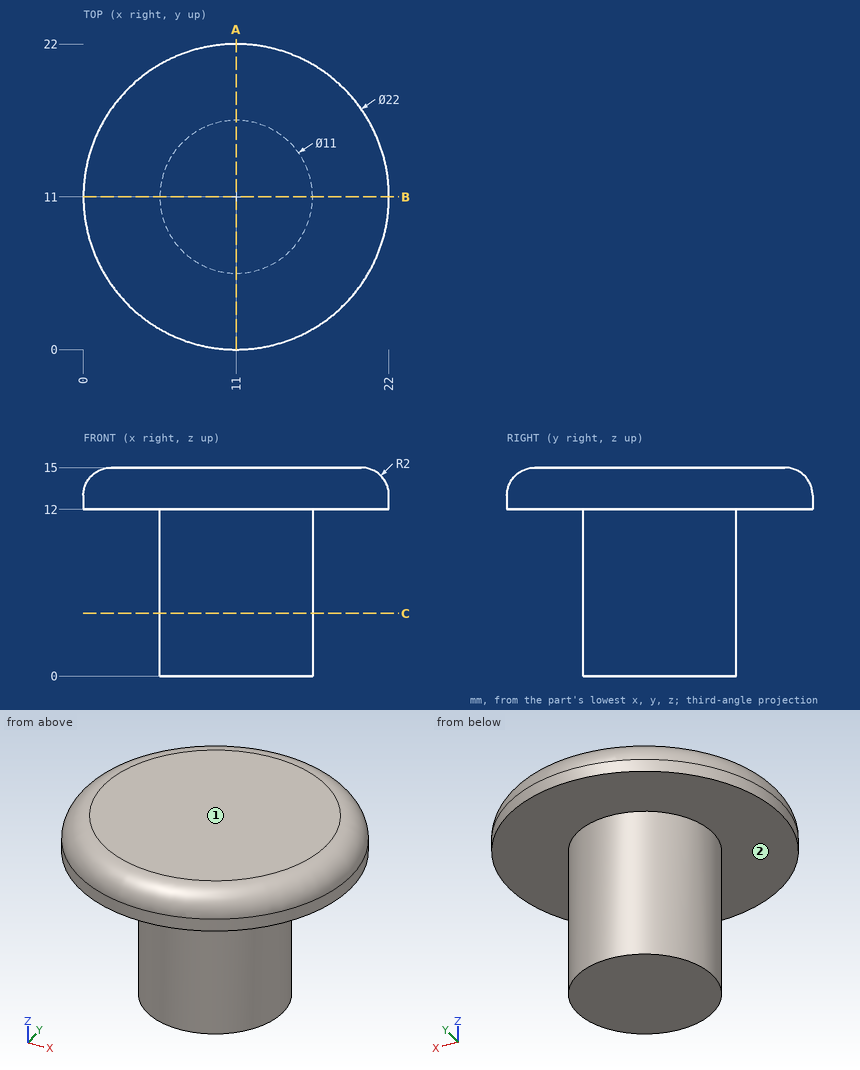
For this review, use the dimensioned drawing (mm, ordinates from the lowest corner) and the shaded views. A direction names the side the tool comes from. Give positions to 0.01 mm unless a question says otherwise; leave off trailing zeros. Loops run counter-clockwise (first coordinate to the right, second up) from the corner with the lowest first, then second, coordinate; pieces in that order, holes last.
Item 1: Take a section at A-A, the plane x = 11. State the section outline as (y, z) points, and give its area (3 significant figures).
Item 2: Tool access review of the marked faces 1 and 2: name each direction out of +Z, -Z, +X, -X, +Y, -Y from which nothing blocks a thin tool from reaching the whole face with its end or side.
Item 3: Insertion check: pin 1 (8 mm diameter, centred on y = 15, z = 4, fed in from -X); pin 2 (4 mm diameter, centred on y = 14, z = 11.5, fed in from -X); pin 3 (1 mm diameter, centred on x = 8.5, z = 7.5, fed in from +Y). Each pin has a flat end and moves straight along its axis. Give the tip position at first contact, or say it passes through.
Item 4: Take a section at C-C, the plane z = 4.5. State the section outline as (x, y) points, and give its area (3 significant figures).
Item 5: For line 1 along Y through (x, z) = (11, 2.75); line 2 along Z through (x, y) = (7.75, 16); line 3 along Y through (x, z) = (15.75, 12.75), list the stretches that pass through material, from the lowest coordinate up.
Calculated:
1. outline: (0, 12) - (5.5, 12) - (5.5, 0) - (16.5, 0) - (16.5, 12) - (22, 12) - (22, 13) arc R2 ccw to (20, 15) - (2, 15) arc R2 ccw to (0, 13) - close
1. area: 196 mm2
2. face 1: +Z, +X, -X, +Y, -Y
2. face 2: -Z
3. pin 1: stops at x = 5.5
3. pin 2: stops at x = 0.05
3. pin 3: stops at y = 16.12
4. outline: circle Ø11 at (11, 11)
4. area: 95.0 mm2
5. line 1: y = 5.5 to 16.5
5. line 2: z = 12 to 15
5. line 3: y = 1.08 to 20.92
